Autodesk Inventor part; units mm, degrees
ref_plane "YZ Plane" through (0, 0, 0) normal (1, 0, 0) x (0, 1, 0)
ref_plane "XZ Plane" through (0, 0, 0) normal (0, 1, 0) x (-1, 0, 0)
ref_plane "XY Plane" through (0, 0, 0) normal (0, 0, 1) x (1, 0, 0)
sketch "Sketch1" plane through (0, 0, 0) normal (0, 1, 0) x (-1, 0, 0)
  line L0 (0, 0) -> (0, -300)
  line L1 (0, -300) -> (-115, -300)
  line L2 (-115, -300) -> (-115, -355)
  line L3 (-115, -355) -> (-230, -355)
  line L4 (-230, -355) -> (-345, -355) construction
  line L5 (0, 0) -> (-345, 0)
  line L6 (-345, 0) -> (-345, -240)
  line L7 (-270, -300) -> (-270, -315)
  line L8 (-345, -240) -> (-270, -300) construction
  line L9 (-307.5, -270) -> (-270, -300) construction
  line L10 (-307.5, -270) -> (-345, -240) construction
  arc A0 (-307.5, -270) -> (-270, -300) centre (-260.624645, -249.843306) ccw
  arc A1 (-307.5, -270) -> (-345, -240) centre (-353.647258, -289.246573) ccw
  arc A2 (-230, -355) -> (-270, -315) centre (-270.80177, -355.80177) ccw
  point P0 (-288.75, -285)
  point P1 (-326.25, -255)
  dimension "d0" = 300
  dimension "d1" = 115
  dimension "d2" = 55
  dimension "d3" = 115
  dimension "d4" = 115
  dimension "d5" = 345
  dimension "d7" = 15
  dimension "d8" = 155
  dimension "d9" = 40
  dimension "d13" = 50
  dimension "d14" = 50
  dimension "d16" = 62.5
  dimension "d19" = 60
extrude "Extrusion1" add sketch "Sketch1" along normal blind 299
sketch "Sketch2" plane through (0, 299, 0) normal (0, 1, 0) x (1, 0, 0)
  line L0 (230, 355) -> (115, 355)
  line L1 (115, 355) -> (115, 300)
  line L2 (115, 300) -> (0, 300)
  line L3 (0, 300) -> (0, 0)
  line L4 (0, 0) -> (345, 0)
  line L5 (345, 0) -> (345, 240)
  arc A0 (307.5, 270) -> (345, 240) centre (353.647258, 289.246573) ccw
  arc A1 (307.5, 270) -> (270, 300) centre (260.624645, 249.843306) ccw
  line L6 (270, 300) -> (270, 315)
  arc A2 (230, 355) -> (270, 315) centre (270.80177, 355.80177) ccw
extrude "Extrusion2" add sketch "Sketch2" along normal blind 1281
sketch "Sketch3" plane through (0, 0, 0) normal (0, -1, 0) x (1, 0, 0)
  line L0 (230, -355) -> (115, -355)
  line L1 (115, -355) -> (115, -300)
  line L2 (115, -300) -> (0, -300)
  line L3 (0, -300) -> (0, 0)
  line L4 (0, 0) -> (345, 0)
  line L5 (345, 0) -> (345, -240)
  line L6 (230, -355) -> (345, -355)
  line L7 (345, -355) -> (345, -240)
extrude "Extrusion3" add sketch "Sketch3" along normal blind 515
sketch "Sketch4" plane through (0, 1580, 0) normal (0, 1, 0) x (1, 0, 0)
  line L0 (345, 0) -> (345, 240)
  line L1 (0, 0) -> (345, 0)
  line L2 (0, 300) -> (0, 0)
  line L3 (115, 300) -> (0, 300)
  line L4 (115, 355) -> (115, 300)
  line L5 (345, 355) -> (345, 240)
  line L6 (345, 240) -> (345, 355)
  line L7 (345, 355) -> (115, 355)
extrude "Extrusion4" add sketch "Sketch4" along normal blind 515
sketch "Sketch5" plane through (0, 1580, 0) normal (0, -1, 0) x (1, 0, 0)
  arc A0 (270, -315) -> (230, -355) centre (270.80177, -355.80177) ccw
  line L0 (345, -355) -> (230, -355)
  line L1 (345, -240) -> (345, -355)
  arc A1 (345, -240) -> (307.5, -270) centre (353.647258, -289.246573) ccw
  arc A2 (270, -300) -> (307.5, -270) centre (260.624645, -249.843306) ccw
  line L2 (270, -300) -> (270, -315)
  line L3 (424.37671, -355) -> (-70.729452, -355)
  point P0 (0, 0)
revolve "Revolution1" cut sketch "Sketch5" angle 360 about axis through (345, 1580, -355) along (-1, 0, 0)
sketch "Sketch6" plane through (0, 0, 0) normal (0, 1, 0) x (1, 0, 0)
  arc A0 (307.5, 270) -> (345, 240) centre (353.647258, 289.246573) ccw
  line L0 (345, 355) -> (345, 240)
  line L1 (230, 355) -> (345, 355)
  arc A1 (230, 355) -> (270, 315) centre (270.80177, 355.80177) ccw
  line L2 (270, 300) -> (270, 315)
  arc A2 (307.5, 270) -> (270, 300) centre (260.624645, 249.843306) ccw
  line L3 (-70.729452, 355) -> (424.37671, 355)
  point P0 (0, 0)
revolve "Revolution2" cut sketch "Sketch6" angle 360 about axis through (115, 0, -355) along (1, 0, 0)
sketch "Sketch12" plane through (345, -515, -355) normal (0, 0, -1) x (-1, 0, 0)
  arc A0 (0, 400) -> (37.5, 430) centre (-8.647258, 449.246573) ccw
  arc A1 (75, 460) -> (37.5, 430) centre (84.375355, 409.843306) ccw
  line L0 (75, 475) -> (75, 460)
  arc A2 (75, 475) -> (115, 515) centre (74.19823, 515.80177) ccw
  line L1 (0, 515) -> (37.5, 515)
  line L2 (75, 515) -> (37.5, 515)
  line L3 (75, 515) -> (115, 515)
  line L4 (0, 400) -> (0, 515)
  point P0 (345, 515)
extrude "Extrusion10" cut sketch "Sketch12" against normal blind 115
sketch "Sketch13" plane through (345, -515, -355) normal (0, 0, -1) x (-1, 0, 0)
  arc A0 (115, 2095) -> (75, 2135) centre (74.19823, 2094.19823) ccw
  line L0 (75, 2150) -> (75, 2135)
  arc A1 (37.5, 2180) -> (75, 2150) centre (84.375355, 2200.156694) ccw
  arc A2 (37.5, 2180) -> (0, 2210) centre (-8.647258, 2160.753427) ccw
  line L1 (0, 2095) -> (0, 2210)
  line L2 (0, 2095) -> (37.5, 2095)
  line L3 (75, 2095) -> (37.5, 2095)
  line L4 (75, 2095) -> (115, 2095)
  point P0 (345, 515)
extrude "Extrusion11" cut sketch "Sketch13" against normal blind 115
sketch "Sketch14" plane through (230, 0, -240) normal (0, -1, 0) x (1, 0, 0)
  arc A0 (40, -75) -> (0, -115) centre (40.80177, -115.80177) ccw
  line L0 (40, -60) -> (40, -75)
  arc A1 (40, -60) -> (77.5, -30) centre (30.624645, -9.843306) ccw
  arc A2 (115, 0) -> (77.5, -30) centre (123.647258, -49.246573) ccw
  line L1 (115, 0) -> (0, 0)
  line L2 (0, -115) -> (0, 0)
  point P0 (-230, 240)
extrude "Extrusion12" add sketch "Sketch14" along normal up to next
sketch "Sketch15" plane through (230, 1580, -240) normal (0, 1, 0) x (1, 0, 0)
  arc A0 (77.5, 30) -> (115, 0) centre (123.647258, 49.246573) ccw
  arc A1 (77.5, 30) -> (40, 60) centre (30.624645, 9.843306) ccw
  line L0 (40, 75) -> (40, 60)
  arc A2 (0, 115) -> (40, 75) centre (40.80177, 115.80177) ccw
  line L1 (0, 115) -> (0, 0)
  line L2 (0, 0) -> (115, 0)
  point P0 (-230, -240)
extrude "Extrusion13" add sketch "Sketch15" along normal up to next
sketch "Sketch16" plane through (0, -515, 0) normal (0, -1, 0) x (1, 0, 0)
  line L0 (0, -300) -> (115, -300)
  line L1 (0, 0) -> (0, -300)
  line L2 (0, 0) -> (115, 0)
  line L3 (115, 0) -> (115, -300)
extrude "Extrusion14" cut sketch "Sketch16" against normal through all
properties part number "Base Drawing"
Geometry: final body of the model. Coordinates: model frame, mm. A direction names the side the tool comes from. Round coordinates to 2 decimals unless told otherwise and drop trailing zeros. Loops run counter-clockwise (first coordinate to the right, second up) from the corner with the lowest first, then second, coordinate; pieces in that order, holes last.
Item 1: Reachability of faces 1 (the flat face through (270, 786, -309)), 2 (the flat face through (206, 772, -355)) from +Z, -Z, +X, -X, +Y, -Y: full face, straight path, thin tool, end or side. Return the list, or none.
Checked values:
face 1: -Z, +X
face 2: -Z, +X, -X, +Y, -Y
Item 2: Section A-A, the plane y = 763.5. Output: boundary loops of the cut face in (x, z), plus the area to 3 significant figures.
Checked values:
outline: (115, -355) - (230, -355) arc R40.81 cw to (270, -315) - (270, -300) arc R51.03 ccw to (307.5, -270) arc R50 cw to (345, -240) - (345, 0) - (115, 0) - close
area: 74,000 mm2
Item 3: Line query: L1, parallel to Z at x = 267, y = 484.5; L2, parallel to Y at x = 291, z = -341; L3, parallel to Y at x = 311, z = -325. Output: solid intervals per line, ascending.
Checked values:
L1: z = -315.17 to 0
L2: y = -515 to -64.16, 1644.16 to 2095
L3: y = -515 to -91.85, 1671.85 to 2095
